```python
from build123d import *

# Parameters (mm, degrees)
ESQUISSE1_W                  = 52.5
ESQUISSE1_H                  = 57.5
ESQUISSE1_W_2                = 42.5
ESQUISSE1_H_2                = 47.5
EXTRU_MINCE1_DEPTH           = 20
ESQUISSE3_W                  = 6.75
ESQUISSE3_H                  = 41
ESQUISSE3_W_2                = 30.75
BOSS_EXTRU_1_DEPTH           = 45
ESQUISSE6_W                  = 5
ESQUISSE6_H                  = 23
ESQUISSE6_W_2                = 13.5
ESQUISSE6_H_2                = 5
BOSS_EXTRU_3_DEPTH           = 5
ENL_V_MAT_EXTRU_1_REACH      = 100.236
ESQUISSE2_R                  = 1.6
ENL_V_START                  = -3
ENL_V_MAT_EXTRU_2_DEPTH      = 3
CONG_1_R                     = 3
ENL_V_MAT_EXTRU_3_DEPTH      = 116.440731547
ENL_V_MAT_EXTRU_4_DEPTH      = 95.578010129
ENL_V_MAT_EXTRU_5_DEPTH      = 85.679173945
ENL_V_MAT_EXTRU_5_DEPTH_BACK = 85.679173945
ESQUISSE11_W                 = 64.25
ESQUISSE11_H                 = 72.384582196


with BuildPart() as part:
    # Esquisse1 → Extru.-Mince1 (new body)
    with BuildSketch(Plane(origin=(0, 0, 0), x_dir=(1, 0, 0), z_dir=(0, 1, 0))):
        Rectangle(ESQUISSE1_W, ESQUISSE1_H)
        Rectangle(ESQUISSE1_W_2, ESQUISSE1_H_2, mode=Mode.SUBTRACT)
    extrude(amount=EXTRU_MINCE1_DEPTH)

    # Esquisse3 → Boss.-Extru.1 (add)
    with BuildSketch(Plane.XZ):
        Polygon((26.25, 28.75), (38, 28.75), (38, -22.25), (21.25, -22.25), (21.25, 23.75), (-21.25, 23.75), (-21.25, -22.25), (-62, -22.25), (-62, 28.75), (-26.25, 28.75), (0, 28.75), align=None)
        with Locations((29.625, 3.25)):
            Rectangle(ESQUISSE3_W, ESQUISSE3_H, mode=Mode.SUBTRACT)
        with Locations((-41.625, 3.25)):
            Rectangle(ESQUISSE3_W_2, ESQUISSE3_H, mode=Mode.SUBTRACT)
    extrude(amount=-BOSS_EXTRU_1_DEPTH)

    # Esquisse6 → Boss.-Extru.3 (add)
    with BuildSketch(Plane(origin=(0, 45, 0), x_dir=(1, 0, 0), z_dir=(0, 1, 0))):
        with Locations((35.5, -5.25)):
            Rectangle(ESQUISSE6_W, ESQUISSE6_H)
        with Locations((16.25, -26.25)):
            Rectangle(ESQUISSE6_W_2, ESQUISSE6_H_2)
        with Locations((-12.25, -26.25)):
            Rectangle(ESQUISSE6_W_2, ESQUISSE6_H_2)
        with Locations((-40.75, -26.25)):
            Rectangle(ESQUISSE6_W_2, ESQUISSE6_H_2)
        with Locations((-40.75, 19.75)):
            Rectangle(ESQUISSE6_W_2, ESQUISSE6_H_2)
        with Locations((-59.5, -5.25)):
            Rectangle(ESQUISSE6_W, ESQUISSE6_H)
    boss_extru_3 = extrude(amount=BOSS_EXTRU_3_DEPTH)

    # Esquisse2 → Enlèv. mat.-Extru.1 (cut, up to next)
    with BuildSketch(Plane.XY.offset(28.75), mode=Mode.PRIVATE) as enl_v_mat_extru_1_sk1:
        with Locations((-15.5, 5.2)):
            Circle(ESQUISSE2_R)
    enl_v_mat_extru_1_tool1 = extrude(enl_v_mat_extru_1_sk1.sketch, amount=-ENL_V_MAT_EXTRU_1_REACH, mode=Mode.PRIVATE) & part.part
    # Esquisse2 → Enlèv. mat.-Extru.1 (cut, up to next)
    with BuildSketch(Plane.XY.offset(28.75), mode=Mode.PRIVATE) as enl_v_mat_extru_1_sk2:
        with Locations((15.5, 5.2)):
            Circle(ESQUISSE2_R)
    enl_v_mat_extru_1_tool2 = extrude(enl_v_mat_extru_1_sk2.sketch, amount=-ENL_V_MAT_EXTRU_1_REACH, mode=Mode.PRIVATE) & part.part
    # Esquisse2 → Enlèv. mat.-Extru.1 (cut, up to next)
    with BuildSketch(Plane.XY.offset(28.75), mode=Mode.PRIVATE) as enl_v_mat_extru_1_sk3:
        with Locations(Location((15.5, 34.8, 0), (0, 0, 180))):
            Circle(ESQUISSE2_R)
    enl_v_mat_extru_1_tool3 = extrude(enl_v_mat_extru_1_sk3.sketch, amount=-ENL_V_MAT_EXTRU_1_REACH, mode=Mode.PRIVATE) & part.part
    # Esquisse2 → Enlèv. mat.-Extru.1 (cut, up to next)
    with BuildSketch(Plane.XY.offset(28.75), mode=Mode.PRIVATE) as enl_v_mat_extru_1_sk4:
        with Locations(Location((-15.5, 34.8, 0), (0, 0, 180))):
            Circle(ESQUISSE2_R)
    enl_v_mat_extru_1_tool4 = extrude(enl_v_mat_extru_1_sk4.sketch, amount=-ENL_V_MAT_EXTRU_1_REACH, mode=Mode.PRIVATE) & part.part
    # Esquisse2 → Enlèv. mat.-Extru.1 (cut, up to next)
    with BuildSketch(Plane.XY.offset(28.75), mode=Mode.PRIVATE) as enl_v_mat_extru_1_sk5:
        with BuildLine():
            Line((2.65, 36.215870824), (2.65, 32.215870824))
            ThreePointArc((2.65, 32.215870824), (0, 7.5), (-2.65, 32.215870824))
            Line((-2.65, 32.215870824), (-2.65, 36.215870824))
            ThreePointArc((-2.65, 36.215870824), (0, 38.865870824), (2.65, 36.215870824))
        make_face()
    enl_v_mat_extru_1_tool5 = extrude(enl_v_mat_extru_1_sk5.sketch, amount=-ENL_V_MAT_EXTRU_1_REACH, mode=Mode.PRIVATE) & part.part
    add(enl_v_mat_extru_1_tool1.solids().sort_by_distance((-15.5, 5.2, 28.75))[0], mode=Mode.SUBTRACT)
    add(enl_v_mat_extru_1_tool2.solids().sort_by_distance((15.5, 5.2, 28.75))[0], mode=Mode.SUBTRACT)
    add(enl_v_mat_extru_1_tool3.solids().sort_by_distance((15.5, 34.8, 28.75))[0], mode=Mode.SUBTRACT)
    add(enl_v_mat_extru_1_tool4.solids().sort_by_distance((-15.5, 34.8, 28.75))[0], mode=Mode.SUBTRACT)
    add(enl_v_mat_extru_1_tool5.solids().sort_by_distance((0, 20.91985, 28.75))[0], mode=Mode.SUBTRACT)

    # Esquisse4 → Enlèv. mat.-Extru.2 (cut)
    with BuildSketch(Plane(origin=(0, 0, 23.75), x_dir=(-1, 0, 0), z_dir=(0, 0, -1)).offset(ENL_V_START)):
        with BuildLine():
            Line((-12.5, 20), (-12.5, 50))
            Line((-12.5, 50), (12.5, 50))
            Line((12.5, 50), (12.5, 20))
            ThreePointArc((12.5, 20), (0, 32.5), (-12.5, 20))
        make_face()
    extrude(amount=ENL_V_MAT_EXTRU_2_DEPTH, mode=Mode.SUBTRACT)

    # Symétrie1: Boss.-Extru.3 across plane
    add(boss_extru_3.mirror(Plane(origin=(0, 22.5, 0), x_dir=(0, 0, 1), z_dir=(0, -1, 0))))

    # Congé1
    cong_1_edges = [part.edges().sort_by_distance(p)[0] for p in [
        (0, 20, -23.75),
    ]]
    fillet(cong_1_edges, radius=CONG_1_R)

    # Esquisse7 → Enlèv. mat.-Extru.3 (cut, through all)
    with BuildSketch(Plane(origin=(38, 0, 0), x_dir=(0, 0, -1), z_dir=(1, 0, 0))):
        with BuildLine():
            Line((-11.75, 38), (5.25, 38))
            ThreePointArc((5.25, 38), (12.321067812, 35.071067812), (15.25, 28))
            Line((15.25, 28), (15.25, 17))
            ThreePointArc((15.25, 17), (12.321067812, 9.928932188), (5.25, 7))
            Line((5.25, 7), (-11.75, 7))
            ThreePointArc((-11.75, 7), (-18.821067812, 9.928932188), (-21.75, 17))
            Line((-21.75, 17), (-21.75, 28))
            ThreePointArc((-21.75, 28), (-18.821067812, 35.071067812), (-11.75, 38))
        make_face()
    extrude(amount=-ENL_V_MAT_EXTRU_3_DEPTH, mode=Mode.SUBTRACT)

    # Esquisse8 → Enlèv. mat.-Extru.4 (cut, through all)
    with BuildSketch(Plane(origin=(0, 0, -22.25), x_dir=(-1, 0, 0), z_dir=(0, 0, -1))):
        with BuildLine():
            Line((48.625, 30), (48.625, 15))
            ThreePointArc((48.625, 15), (41.625, 8), (34.625, 15))
            Line((34.625, 15), (34.625, 30))
            ThreePointArc((34.625, 30), (41.625, 37), (48.625, 30))
        make_face()
    extrude(amount=-ENL_V_MAT_EXTRU_4_DEPTH, mode=Mode.SUBTRACT)

    # Esquisse11 → Enlèv. mat.-Extru.5 (cut, two sides: drawn at the far end of the back side and taken through both)
    with BuildSketch(Plane(origin=(0, 45, 0), x_dir=(1, 0, 0), z_dir=(0, 1, 0)).offset(-ENL_V_MAT_EXTRU_5_DEPTH_BACK)):
        with Locations((5.875, 7.442291098)):
            Rectangle(ESQUISSE11_W, ESQUISSE11_H)
    extrude(amount=ENL_V_MAT_EXTRU_5_DEPTH + ENL_V_MAT_EXTRU_5_DEPTH_BACK, mode=Mode.SUBTRACT)


solid = part.part
```
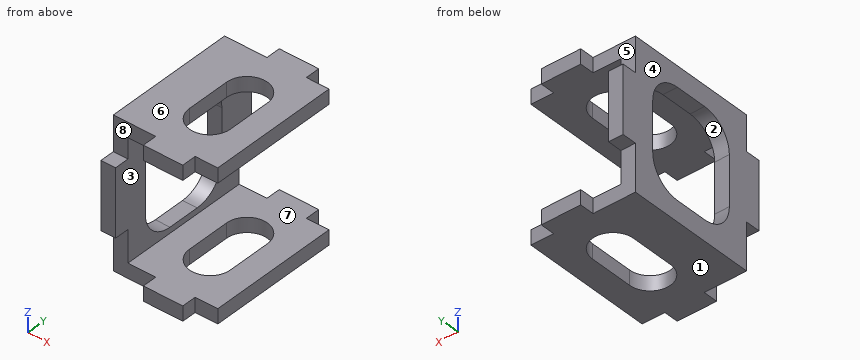
Geometry: final body of the model. Coordinates: model frame, mm. Face numbers are marked on the shaded views. A direction names the side the tool comes from. Coordinates: 2 decimals unless noted, no trailing zeros. Order: outer loops, then holes, each group sorted by start corner. A loop starts at its lowest first (then second) coordinate and runs counter-clockwise, first axis right, second up. Notation, with made-up numbers: (75, 43.5) - (133, 43.5) arc R26 ccw to (133, 66.5) - close; hole circle Ø4 at (71.25, 41). An arc over 180 degrees is marked (long way). Write each question's results on one line, items separated by ' | '.
(1) Mould query, pull axis Z, two halves, no side actions, for the marked faces 6, 7 and 8. Classes: +Z half, -Z half, draft (parallel to the pull), parting line (faces both ways), or undercut.
Values found:
face 6: +Z half | face 7: undercut | face 8: draft
(2) First-contact query: pin 1 Ø5.5 at (x, z) = (-31, 26) entering from -Y; pin 2 Ø6 at (y, z) = (44, 10.5) entering from +X; pin 3 Ø2.5 at (x, y) = (-60, -3) entering from -Z; pin 4 Ø4 at (x, z) = (-56, -0.5) entering from +Y. Flat tips, straight axial feed; report the tip coordinate or a pass-through.
Values found:
pin 1: stops at y = 0 | pin 2: stops at x = -57 | pin 3: stops at z = -6.25 | pin 4: stops at y = 50
(3) Section query B-B, the plane y = 32. Return the cut outline in (x, z), plus the area to 3 significant figures.
Values found:
outline: (-62, -22.25) - (-48.33, -22.25) - (-48.33, -17.25) - (-57, -17.25) - (-57, -14.42) - (-62, -14.42) - close; (-62, 20.92) - (-57, 20.92) - (-57, 23.75) - (-48.33, 23.75) - (-48.33, 28.75) - (-62, 28.75) - close; (-34.92, -22.25) - (-26.25, -22.25) - (-26.25, -17.25) - (-34.92, -17.25) - close; (-34.92, 23.75) - (-26.25, 23.75) - (-26.25, 28.75) - (-34.92, 28.75) - close | area: 252 mm²
(4) Section query D-D, the plane y = 10.5. Return the cut outline in (x, z), plus the area to 3 significant figures.
Values found:
outline: (-62, -22.25) - (-46.99, -22.25) - (-46.99, -17.25) - (-57, -17.25) - (-57, -12.85) - (-62, -12.85) - close; (-62, 19.35) - (-57, 19.35) - (-57, 23.75) - (-46.99, 23.75) - (-46.99, 28.75) - (-62, 28.75) - close; (-36.26, -22.25) - (-26.25, -22.25) - (-26.25, -17.25) - (-36.26, -17.25) - close; (-36.26, 23.75) - (-26.25, 23.75) - (-26.25, 28.75) - (-36.26, 28.75) - close | area: 294 mm²
(5) Set-up query: the marked faces 1, 2, 3, 4 and 5. Return all of +Z, -Z, +X, -X, +Y, -Y with unobstructed straight access to the full face (end or side cutting, diameter ignored); none if empty.
Values found:
face 1: -Z, +X, -X, +Y, -Y | face 2: +X, -X | face 3: +X, +Y, -Y | face 4: +Z, -Z, -X, +Y, -Y | face 5: +Z, -X, +Y
(6) Section query A-A, the plane x = -59. Return the cut outline in (y, z).
Values found:
outline: (-5, -6.25) - (0, -6.25) - (0, -22.25) - (45, -22.25) - (45, -6.25) - (50, -6.25) - (50, 16.75) - (45, 16.75) - (45, 28.75) - (0, 28.75) - (0, 16.75) - (-5, 16.75) - close; hole (7, -5.25) arc R10 ccw to (17, -15.25) - (28, -15.25) arc R10 ccw to (38, -5.25) - (38, 11.75) arc R10 ccw to (28, 21.75) - (17, 21.75) arc R10 ccw to (7, 11.75) - close
(7) Line query: line 1 (Z direction, x = -55, y = 23); line 2 (X direction, y = 42, z = -15); line 3 (X direction, y = 47.5, z = 25). Output: solid intervals per line, ascending. Write a range as [from, to].
Values found:
line 1: z = [-22.25, -17.25], [23.75, 28.75] | line 2: x = [-62, -57] | line 3: x = [-47.5, -34]
(8) Section query C-C, the plane y = 2. Return the cut outline in (x, z).
Values found:
outline: (-62, -22.25) - (-26.25, -22.25) - (-26.25, -17.25) - (-57, -17.25) - (-57, 23.75) - (-26.25, 23.75) - (-26.25, 28.75) - (-62, 28.75) - close
